Design review of the part built by this model. Coordinates are the model's own, in mm. A direction names the side the tool comes from. Coordinates: 2 decimals unless noted, no trailing zeros. Loops run counter-clockwise (first coordinate to the right, second up) from the corner with the lowest first, then second, coordinate; pieces in that order, holes last. Notation, with made-up numbers: (-6.5, 33.5) -> (27.5, 33.5) arc R21 ccw to (27.5, 41.5) -> close; hole circle Ø6 at (-37.5, 56.5). An arc over 180 degrees is marked (long way). Use a Markdown table: item, result. Add a question column.
Q1. Clearance check with flat-ended pins moving along their axes: pin 1 Ø15 at (y, z) = (-22.5, 11) entering from +X; pin 2 Ø9 at (y, z) = (-18, 8.5) entering from -X; pin 3 Ø1 at (y, z) = (-91, 22) entering from -X. State where each tip first meets the part, or that it passes through.
Q2. For faces 4 (the face through (15, -34, 15)), 5 (the face through (11, 15, 15)), 6 (the face through (4, 0, 15)), 7 (the face through (-7, -36, 15)), list the 3-axis set-ups (+Z, -Z, +X, -X, +Y, -Y) from which the entire face can be reached by the end or side of a thin tool; tool diameter is ignored.
Q3. Take a section at B-B on x = 6.5. Write out the cut boundary in (y, z), plus the area to 3 significant figures.
Q4. Take a section at A-A on z = 10.5. Write out the cut boundary in (x, y).
Q5. For probe 1 along X at (y, z) = (3, 3); probe 2 along X at (y, z) = (-20.5, 12.5); probe 3 along Y at (x, z) = (-21.5, 10.5), list the stretches that pass through material, from the lowest coordinate up.
Q6. Draft analysis for pull direction X (two halves, no side actions). For faces 1 (the face through (-17, -95, 15)), 2 (the face through (-4, 15, 15)), 3 (the face through (0, 8, 15)), state which applies: pulls with the +X half, pulls with the -X half, needs draft (parallel to the pull), parting line crosses it, or undercut.
Q7. Take a section at C-C on y = -36.5. Write out the cut boundary in (x, z), plus the area to 3 significant figures.
from build123d import *

# Parameters (mm, degrees)
BOSS_EXTRUDE1_DEPTH = 30
BOSS_EXTRUDE2_DEPTH = 30


with BuildPart() as part:
    # Sketch1 → Boss-Extrude1 (new body)
    with BuildSketch(Plane.XY):
        Polygon((0, 0), (8, 0), (8, 15), (15, 15), (15, -105), (-7, -105), (-7, 15), (0, 15), align=None)
    extrude(amount=BOSS_EXTRUDE1_DEPTH)

    # Sketch2 → Boss-Extrude2 (add)
    with BuildSketch(Plane.XY.offset(30)):
        Polygon((15, -85), (35, -105), (15, -105), align=None)
    boss_extrude2 = extrude(amount=-BOSS_EXTRUDE2_DEPTH)

    # Mirror1: Boss-Extrude2 across plane
    add(boss_extrude2.mirror(Plane.ZY.offset(-4)))


solid = part.part
Answer list:
| question | item | result |
|---|---|---|
| 1 | pin 1 | x = 15 |
| 1 | pin 2 | x = -7 |
| 1 | pin 3 | x = -13.5 |
| 2 | face 4 | +Z, -Z, +X, +Y |
| 2 | face 5 | +Z, -Z, +X, -X, +Y |
| 2 | face 6 | +Z, -Z, +Y |
| 2 | face 7 | +Z, -Z, -X, +Y |
| 3 | outline | (-105, 0) -> (0, 0) -> (0, 30) -> (-105, 30) -> close |
| 3 | area | 3,150 mm² |
| 4 | outline | (-27, -105) -> (35, -105) -> (15, -85) -> (15, 15) -> (8, 15) -> (8, 0) -> (0, 0) -> (0, 15) -> (-7, 15) -> (-7, -85) -> close |
| 5 | probe 1 | -7 to 0, 8 to 15 |
| 5 | probe 2 | -7 to 15 |
| 5 | probe 3 | -105 to -99.5 |
| 6 | face 1 | pulls with the -X half |
| 6 | face 2 | needs draft |
| 6 | face 3 | undercut |
| 7 | outline | (-7, 0) -> (15, 0) -> (15, 30) -> (-7, 30) -> close |
| 7 | area | 660 mm² |
